Source: three-view drawing plus pictorial views. Frame: mm from the lowest corner of the part. Round coordinates to 2 decimals unless told otherwise and drop trailing zeros. Write each loop counter-clockwise with the first axis right and the second up, starting at its lowest first coordinate (ties: lowest second). Pieces come first, ordered by that corner, then holes. Notation, with made-up numbers: M -37.75,-25.5 L 12.25,-25.5 A13 cw 12.25,-17.5 Z; hole C 72.5,-30 d2. An arc over 180 degrees is marked long. Answer in a Markdown table with one row per item.
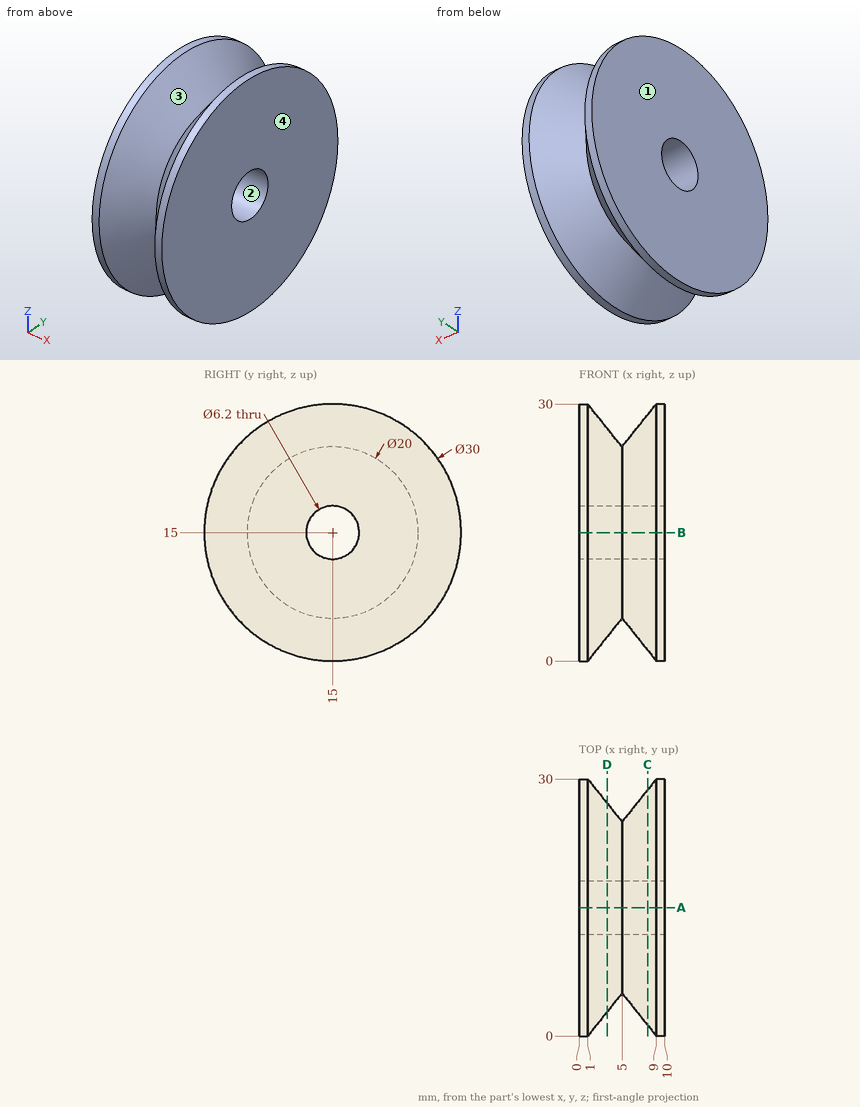
Q1. Contact query for flat-ended pins moving along their axis: pin 1 Ø6 at (x, z) = (5, 8.5) entering from -Y; pin 2 Ø5 at (x, y) = (4.5, 17) entering from -Z; pin 3 Ø4 at (x, y) = (4.5, 25) entering from +Z. Output: stop coordinate, or through.
Solutions:
| item | result |
|---|---|
| pin 1 | stops at y = 2.63 |
| pin 2 | stops at z = 1.38 |
| pin 3 | stops at z = 24.09 |
Q2. Pull-direction query (X, two-part tool) for the marked faces 1, 2, 3 and 4; classes: pulls with the +X half, pulls with the -X half, needs draft (parallel to the pull), parting line crosses it, or undercut.
Solutions:
| item | result |
|---|---|
| face 1 | pulls with the -X half |
| face 2 | needs draft |
| face 3 | undercut |
| face 4 | pulls with the +X half |
Q3. Section C-C (x = 8). Return loops of the section in (y, z), and give its area (3 significant figures).
Solutions:
| item | result |
|---|---|
| outline | C 15,15 d27.5; hole C 15,15 d6.2 |
| area | 564 mm2 |
Q4. Section A-A (y = 15). Return loops of the section in (x, z), and give its area (3 significant figures).
Solutions:
| item | result |
|---|---|
| outline | M 0,0 L 1,0 L 5,5 L 9,0 L 10,0 L 10,11.9 L 0,11.9 Z; M 0,18.1 L 10,18.1 L 10,30 L 9,30 L 5,25 L 1,30 L 0,30 Z |
| area | 198 mm2 |
Q5. Section D-D (x = 3.25). Return loops of the section in (y, z) (1 decimal), and give its area (3 significant figures).
Solutions:
| item | result |
|---|---|
| outline | C 15,15 d24.4; hole C 15,15 d6.2 |
| area | 436 mm2 |
Q6. Material intervals for probe 1 along Y at (x, z) = (3, 15); probe 2 along X at (y, z) = (6, 8.25); probe 3 along X at (y, z) = (15, 28.25), sorted ascending.
Solutions:
| item | result |
|---|---|
| probe 1 | y = 2.5 to 11.9, 18.1 to 27.5 |
| probe 2 | x = 0 to 4, 6 to 10 |
| probe 3 | x = 0 to 2.4, 7.6 to 10 |
